For this review, take the finished solid that the model builds, in its own axes (mm). Give positions to 0.01 mm unless a question says otherwise; leave off trailing zeros. Order: outer loops, then holes, each group sorted by start corner. A loop starts at its lowest first (then second) coordinate and runs counter-clockwise, first axis right, second up. Notation, with made-up numbers: (27, 42.5) - (57, 42.5) arc R18 ccw to (57, 74.5) - close; hole circle Ø3 at (-33, 52). An arc over 180 degrees is marked (long way). Put each result on its own line as item: value. Start each with the question number.
```python
from build123d import *

# Parameters (mm, degrees)
SKETCH1_R           = 22
SKETCH1_R_2         = 11.5
SKETCH1_R_3         = 1.65
BOSS_EXTRUDE1_DEPTH = 2.5
BOSS_EXTRUDE2_DEPTH = 4
CHAMFER1_SIZE       = 0.75


with BuildPart() as part:
    # Sketch1 → Boss-Extrude1 (new body)
    with BuildSketch(Plane.XY):
        Circle(SKETCH1_R)
        Circle(SKETCH1_R_2, mode=Mode.SUBTRACT)
        with Locations((0, 17.5)):
            Circle(SKETCH1_R_3, mode=Mode.SUBTRACT)
        with Locations((15.155444566, -8.75)):
            Circle(SKETCH1_R_3, mode=Mode.SUBTRACT)
        with Locations((-15.155444566, -8.75)):
            Circle(SKETCH1_R_3, mode=Mode.SUBTRACT)
    extrude(amount=BOSS_EXTRUDE1_DEPTH)

    # Sketch2 → Boss-Extrude2 (add)
    # profile 1 of 3: a face of its own
    with BuildSketch(Plane.XY.offset(2.5)):
        with BuildLine():
            ThreePointArc((4.426906369, 21.55), (0, 22), (-4.426906369, 21.55))
            ThreePointArc((-4.426906369, 21.55), (0, 11.5), (4.426906369, 21.55))
        make_face()
        Polygon((1.659882024, 20.375), (3.319764048, 17.5), (1.659882024, 14.625), (-1.659882024, 14.625), (-3.319764048, 17.5), (-1.659882024, 20.375), align=None, mode=Mode.SUBTRACT)
    # profile 2 of 3: a face of its own
    with BuildSketch(Plane.XY.offset(2.5)):
        with BuildLine():
            ThreePointArc((-16.449394267, -14.608813376), (-9.959292144, -5.75), (-20.876300636, -6.941186624))
            ThreePointArc((-20.876300636, -6.941186624), (-19.052558883, -11), (-16.449394267, -14.608813376))
        make_face()
        Polygon((-18.475208614, -8.75), (-16.81532659, -5.875), (-13.495562542, -5.875), (-11.835680518, -8.75), (-13.495562542, -11.625), (-16.81532659, -11.625), align=None, mode=Mode.SUBTRACT)
    # profile 3 of 3: a face of its own
    with BuildSketch(Plane.XY.offset(2.5)):
        with BuildLine():
            ThreePointArc((16.449394267, -14.608813376), (19.052558883, -11), (20.876300636, -6.941186624))
            ThreePointArc((20.876300636, -6.941186624), (9.959292144, -5.75), (16.449394267, -14.608813376))
        make_face()
        Polygon((16.81532659, -11.625), (13.495562542, -11.625), (11.835680518, -8.75), (13.495562542, -5.875), (16.81532659, -5.875), (18.475208614, -8.75), align=None, mode=Mode.SUBTRACT)
    extrude(amount=BOSS_EXTRUDE2_DEPTH)

    # Chamfer1
    chamfer1_edges = [part.edges().sort_by_distance(p)[0] for p in [
        (2.489823036, 16.0625, 6.5),
        (0, 14.625, 6.5),
        (-2.489823036, 16.0625, 6.5),
        (-2.489823036, 18.9375, 6.5),
        (2.489823036, 18.9375, 6.5),
        (-15.155444566, -5.875, 6.5),
        (-12.66562153, -7.3125, 6.5),
        (-12.66562153, -10.1875, 6.5),
        (-15.155444566, -11.625, 6.5),
        (-17.645267602, -7.3125, 6.5),
        (12.66562153, -10.1875, 6.5),
        (12.66562153, -7.3125, 6.5),
        (15.155444566, -5.875, 6.5),
        (17.645267602, -7.3125, 6.5),
        (15.155444566, -11.625, 6.5),
    ]]
    chamfer(chamfer1_edges, length=CHAMFER1_SIZE)


solid = part.part
```
1. Add section B-B, the plane y = 0. Give the boundary of the cut face in (x, z), then the cut area to 3 significant figures.
2. Add section C-C, the plane y = 4.5. Give the boundary of the cut face in (x, z).
3. Clearance check with flat-ended pins moving along their axes: pin 1 (12 mm diameter, centred on x = 7.5, y = 2, fed in from +Z); pin 2 (2 mm diameter, centred on x = 0, z = 5.5, fed in from -Y); pin 3 (1 mm diameter, centred on x = 15, z = 4, fed in from +Y). State where each tip first meets the part, or that it passes through.
4. Add section A-A, the plane z = 3.5. Give the boundary of the cut face in (x, y) (3 decimals), then the cut area to 3 significant figures.
5. The part is to be moulded in two halves that separate along X. For faces 1 (the face through (-0.194, 11.503, 4.472)), 2 (the face through (-9.865, -5.92, 4.472)), 3 (the face through (-12, -6, 6.5)), say which applies: released by +X, released by -X, zero draft, split by the parting line, or undercut.
6. Wall thickness on line 1 (Y direction, x = 0, z = 1.75); line 2 (X direction, y = 0, z = 2); line 3 (X direction, y = -9.5, z = 3.75): over which ranges is each line inside the solid? List them lowest first. Write a range as from..to.
Found:
1. outline: (-22, 0) - (-11.5, 0) - (-11.5, 2.5) - (-22, 2.5) - close; (11.5, 0) - (22, 0) - (22, 2.5) - (11.5, 2.5) - close
1. area: 52.5 mm^2
2. outline: (-21.53, 0) - (-10.58, 0) - (-10.58, 2.5) - (-21.53, 2.5) - close; (10.58, 0) - (21.53, 0) - (21.53, 2.5) - (10.58, 2.5) - close
3. pin 1: stops at z = 2.5
3. pin 2: stops at y = 11.5
3. pin 3: stops at y = -2.75
4. outline: (-20.876, -6.941) arc R22 ccw to (-16.449, -14.609) arc R6 ccw (long way) to start; (-4.427, 21.55) arc R6 ccw (long way) to (4.427, 21.55) arc R22 ccw to start; (16.449, -14.609) arc R22 ccw to (20.876, -6.941) arc R6 ccw (long way) to start; hole (-18.475, -8.75) - (-16.815, -11.625) - (-13.496, -11.625) - (-11.836, -8.75) - (-13.496, -5.875) - (-16.815, -5.875) - close; hole (-3.32, 17.5) - (-1.66, 14.625) - (1.66, 14.625) - (3.32, 17.5) - (1.66, 20.375) - (-1.66, 20.375) - close; hole (11.836, -8.75) - (13.496, -11.625) - (16.815, -11.625) - (18.475, -8.75) - (16.815, -5.875) - (13.496, -5.875) - close
4. area: 226 mm^2
5. face 1: split by the parting line
5. face 2: undercut
5. face 3: zero draft
6. line 1: y = -22..-11.5, 11.5..15.85, 19.15..22
6. line 2: x = -22..-11.5, 11.5..22
6. line 3: x = -19.84..-18.04, -12.27..-9.2, 9.2..12.27, 18.04..19.84
